For this review, use the dimensioned drawing (mm, ordinates from the lowest corner) and the shaded views. A direction names the side the tool comes from. Round coordinates to 2 decimals unless told otherwise and drop trailing zeros. Write each loop counter-clockwise with the first axis right and the second up, starting at its lowest first coordinate (ties: lowest second). Pieces come first, ordered by that corner, then holes. Notation, with made-up numbers: (80, -25.75) -> (95, -25.75) arc R15 cw to (95, -11.75) -> close; hole circle Ø7 at (14, -29). An arc over 180 degrees is marked (long way). Answer as CSV lines item,"result". Start each with the question number.
Item 1: Take a section at A-A on x = 9. Give the boundary of the cut face in (y, z), then the cut area to 3 significant figures.
Item 2: Machinability: for the marked faces 4, 5, 6, 7 and 8, which of the approach directions +Z, -Z, +X, -X, +Y, -Y give a long, thin tool a straight path to every point of the face, cutting with its end or side? Answer none if there is none.
Item 3: For pin 1 Ø2.5 at (x, y) = (9, 4.5) entering from +Z; pin 2 Ø1.8 at (x, z) = (9, 9) entering from +Y; pin 3 Ø2.5 at (y, z) = (3.5, 7) entering from -X; pin 4 Ø4 at (x, z) = (10.5, 12) entering from -Y, all flat-tipped, find the tip position at first contact; note any pin that passes through.
Item 4: Take a section at C-C on z = 9. Give the boundary of the cut face in (x, y).
Item 5: Take a section at B-B on y = 4.95. Give the boundary of the cut face in (x, z).
Item 6: Wall thickness on probe 1 along Z at (x, y) = (9, 0.2); probe 2 along X at (y, z) = (4.5, 7.75): over which ranges is each line inside the solid? List them lowest first. Write a range as from..to.
Item 7: Mouldability with a two-part tool opening along Z and no side actions: class the marked faces 1, 2 and 3 as +Z half, -Z half, draft (parallel to the pull), parting line (faces both ways), or undercut.
Item 8: Take a section at D-D on z = 7. Give the boundary of the cut face in (x, y), then the cut area to 3 significant figures.
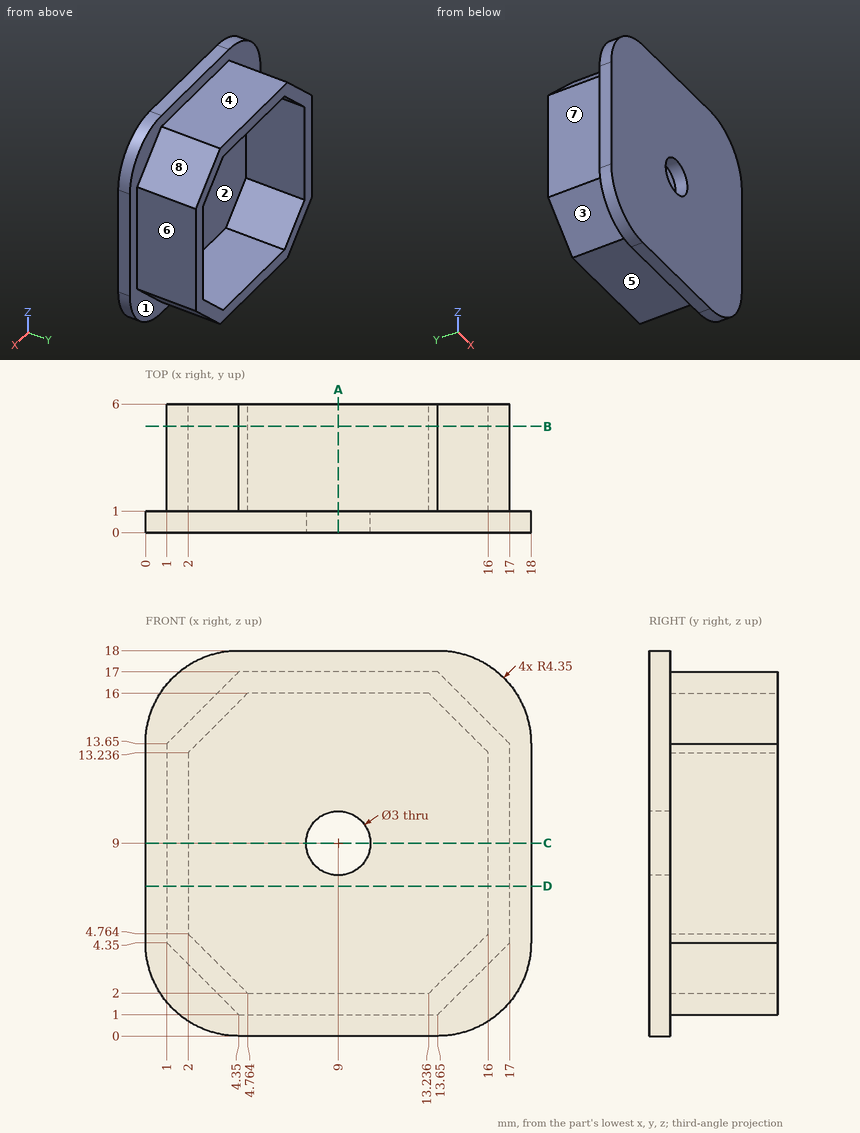
Output values:
1,outline,"(0, 0) -> (1, 0) -> (1, 1) -> (6, 1) -> (6, 2) -> (1, 2) -> (1, 7.5) -> (0, 7.5) -> close; (0, 10.5) -> (1, 10.5) -> (1, 16) -> (6, 16) -> (6, 17) -> (1, 17) -> (1, 18) -> (0, 18) -> close"
1,area,"25.0 mm^2"
2,face 4,"+Z, +X, -X, +Y"
2,face 5,"-Z, +X, -X, +Y"
2,face 6,"+Z, -Z, +X, +Y"
2,face 7,"+Z, -Z, -X, +Y"
2,face 8,"+Z, +X, +Y"
3,pin 1,"stops at z = 17"
3,pin 2,"passes through"
3,pin 3,"stops at x = 1"
3,pin 4,"stops at y = 0"
4,outline,"(0, 0) -> (7.5, 0) -> (7.5, 1) -> (2, 1) -> (2, 6) -> (1, 6) -> (1, 1) -> (0, 1) -> close; (10.5, 0) -> (18, 0) -> (18, 1) -> (17, 1) -> (17, 6) -> (16, 6) -> (16, 1) -> (10.5, 1) -> close"
5,outline,"(1, 4.35) -> (4.35, 1) -> (13.65, 1) -> (17, 4.35) -> (17, 13.65) -> (13.65, 17) -> (4.35, 17) -> (1, 13.65) -> close; hole (2, 4.76) -> (4.76, 2) -> (13.24, 2) -> (16, 4.76) -> (16, 13.24) -> (13.24, 16) -> (4.76, 16) -> (2, 13.24) -> close"
6,probe 1,"z = 0..7.5, 10.5..18"
6,probe 2,"x = 1..2, 16..17"
7,face 1,"draft"
7,face 2,"undercut"
7,face 3,"-Z half"
8,outline,"(0, 0) -> (18, 0) -> (18, 1) -> (17, 1) -> (17, 6) -> (16, 6) -> (16, 1) -> (2, 1) -> (2, 6) -> (1, 6) -> (1, 1) -> (0, 1) -> close"
8,area,"28.0 mm^2"
